Geometry: final body of the model. Coordinates: model frame, mm. Face numbers are marked on the shaded views. Round coordinates to 2 decimals unless told otherwise and drop trailing zeros. Loops run counter-clockwise (first coordinate to the right, second up) from the corner with the lowest first, then second, coordinate; pieces in that order, holes last. Notation, with made-up numbers: (35, -20.5) - (77, -20.5) arc R7 cw to (77, -13.5) - close; hole circle Ø2 at (73, 76.25). An arc over 180 degrees is marked (long way). Answer in a Markdown table with one row per item. Add a question column.
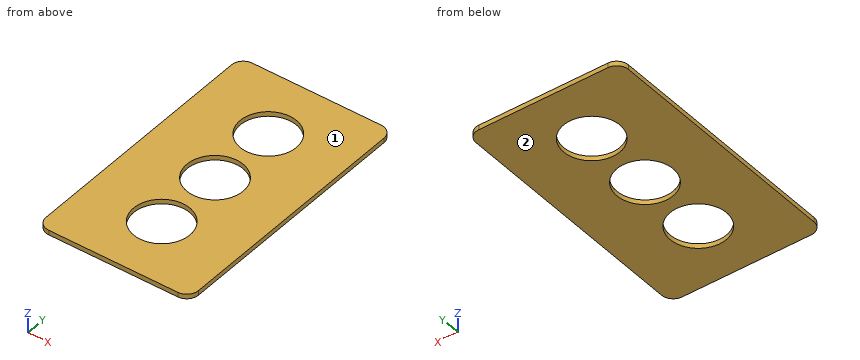
from build123d import *

# Parameters (mm, degrees)
F0_W     = 65
F0_H     = 113.4
F0_R     = 12
F1_DEPTH = 2
F2_R     = 5


with BuildPart() as f1:
    # F0 (on Top) → F1 (new body)
    with BuildSketch(Plane.XY):
        Rectangle(F0_W, F0_H)
        with Locations((0, -29.7)):
            Circle(F0_R, mode=Mode.SUBTRACT)
        Circle(F0_R, mode=Mode.SUBTRACT)
        with Locations((0, 29.7)):
            Circle(F0_R, mode=Mode.SUBTRACT)
    extrude(amount=F1_DEPTH)

    # F2
    f2_edges = [f1.edges().sort_by_distance(p)[0] for p in [
        (-32.5, 56.7, 1),
        (32.5, 56.7, 1),
        (32.5, -56.7, 1),
        (-32.5, -56.7, 1),
    ]]
    fillet(f2_edges, radius=F2_R)


solid = f1.part
1) Section D-D, the plane y = -7. Return the cut outline in (x, z), and give its area (3 significant figures).
2) Section A-A, the plane x = 0. Return the cut outline in (y, z), and give its area (3 significant figures).
3) Section B-B, the plane y = 29.7. Return the cut outline in (x, z).
4) Pull-direction query (Z, two-part tool) for the marked faces 1 and 2; classes: pulls with the +Z half, pulls with the -Z half, needs draft (parallel to the pull), parting line crosses it, or undercut.
5) Section C-C, the plane z = 1.05. Return the cut outline in (x, y), and give its area (3 significant figures).
6) Contact query for a flat-ended pin moving along its axis: pin 1 Ø19 at (x, y) = (0, -29.7) entering from +Z. Output: stop coordinate, or through.
7) Material intervals for line 1 along Y through (x, z) = (0, 0.5); line 2 along Y through (x, z) = (2.5, 0.5); line 3 along X through (y, z) = (-28, 0.7), sorted ascending. Write a range as from..to.
Evaluation:
| question | item | result |
|---|---|---|
| 1 | outline | (-32.5, 0) - (-9.75, 0) - (-9.75, 2) - (-32.5, 2) - close; (9.75, 0) - (32.5, 0) - (32.5, 2) - (9.75, 2) - close |
| 1 | area | 91.0 mm² |
| 2 | outline | (-56.7, 0) - (-41.7, 0) - (-41.7, 2) - (-56.7, 2) - close; (-17.7, 0) - (-12, 0) - (-12, 2) - (-17.7, 2) - close; (12, 0) - (17.7, 0) - (17.7, 2) - (12, 2) - close; (41.7, 0) - (56.7, 0) - (56.7, 2) - (41.7, 2) - close |
| 2 | area | 82.8 mm² |
| 3 | outline | (-32.5, 0) - (-12, 0) - (-12, 2) - (-32.5, 2) - close; (12, 0) - (32.5, 0) - (32.5, 2) - (12, 2) - close |
| 4 | face 1 | pulls with the +Z half |
| 4 | face 2 | pulls with the -Z half |
| 5 | outline | (-32.5, -51.7) arc R5 ccw to (-27.5, -56.7) - (27.5, -56.7) arc R5 ccw to (32.5, -51.7) - (32.5, 51.7) arc R5 ccw to (27.5, 56.7) - (-27.5, 56.7) arc R5 ccw to (-32.5, 51.7) - close; hole circle Ø24 at (0, -29.7); hole circle Ø24 at (0, 0); hole circle Ø24 at (0, 29.7) |
| 5 | area | 5,990 mm² |
| 6 | pin 1 | passes through |
| 7 | line 1 | y = -56.7..-41.7, -17.7..-12, 12..17.7, 41.7..56.7 |
| 7 | line 2 | y = -56.7..-41.44, -17.96..-11.74, 11.74..17.96, 41.44..56.7 |
| 7 | line 3 | x = -32.5..-11.88, 11.88..32.5 |
